The listing builds one solid part. Answer for the finished solid, in the listing's coordinates (mm). Face numbers are marked on the shaded views. A direction names the side the tool comes from. Round coordinates to 2 decimals unless told otherwise and drop trailing zeros. Loops run counter-clockwise (first coordinate to the right, second up) from the corner with the lowest first, then second, coordinate; pieces in that order, holes last. Notation, with made-up numbers: M 38,43.5 L 52,43.5 A14 cw 52,57.5 Z; hole C -12,64 d6. An arc over 180 degrees is marked long. Answer as a JSON object with one key per item and string values.
```python
from build123d import *

# Parameters (mm, degrees)
SKETCH1_W           = 70
SKETCH1_H           = 100
BOSS_EXTRUDE1_DEPTH = 40
SKETCH2_W           = 66
SKETCH2_H           = 92
CUT_EXTRUDE1_DEPTH  = 33
SKETCH3_W           = 4
SKETCH3_H           = 92
CUT_EXTRUDE2_DEPTH  = 71
SKETCH4_R           = 10.75
CUT_EXTRUDE3_DEPTH  = 3.5
CUT_EXTRUDE4_DEPTH  = 5.5
SKETCH6_R           = 1.1
CUT_EXTRUDE5_DEPTH  = 3
SKETCH11_W          = 10
SKETCH11_H          = 92
CUT_EXTRUDE9_DEPTH  = 10
SKETCH12_W          = 2.25
SKETCH12_H          = 40
CUT_EXTRUDE10_DEPTH = 5
SKETCH13_W          = 2.25
SKETCH13_H          = 40
CUT_EXTRUDE11_DEPTH = 5
SKETCH16_R          = 11.75
BOSS_EXTRUDE3_DEPTH = 8.5
SKETCH17_R          = 10.7
CUT_EXTRUDE13_DEPTH = 10
SKETCH19_W          = 20.5
SKETCH19_H          = 10.2
CUT_EXTRUDE14_DEPTH = 101


with BuildPart() as part:
    # Sketch1 → Boss-Extrude1 (new body)
    with BuildSketch(Plane.XY):
        Rectangle(SKETCH1_W, SKETCH1_H)
    extrude(amount=BOSS_EXTRUDE1_DEPTH)

    # Sketch2 → Cut-Extrude1 (cut)
    with BuildSketch(Plane.XY.offset(40)):
        Rectangle(SKETCH2_W, SKETCH2_H)
    extrude(amount=-CUT_EXTRUDE1_DEPTH, mode=Mode.SUBTRACT)

    # Sketch3 → Cut-Extrude2 (cut, through all)
    with BuildSketch(Plane.ZY.offset(35)):
        with Locations((6.5, 0)):
            Rectangle(SKETCH3_W, SKETCH3_H)
    extrude(amount=-CUT_EXTRUDE2_DEPTH, mode=Mode.SUBTRACT)

    # Sketch4 → Cut-Extrude3 (cut)
    with BuildSketch(Plane(origin=(0, 0, 0), x_dir=(-1, 0, 0), z_dir=(0, 0, -1))):
        Circle(SKETCH4_R)
    extrude(amount=-CUT_EXTRUDE3_DEPTH, mode=Mode.SUBTRACT)

    # Sketch5 → Cut-Extrude4 (cut, through all)
    with BuildSketch(Plane.XY.offset(4.5)):
        Polygon((-15.010107583, -6), (-35.010107583, -6), (-35.010107583, 6), (-28.010107583, 6), (-22.010107583, 6), (-15.010107583, 6), align=None)
        Polygon((15.010107583, -6), (35.010107583, -6), (35.010107583, 6), (28.010107583, 6), (22.010107583, 6), (15.010107583, 6), align=None)
    extrude(amount=-CUT_EXTRUDE4_DEPTH, mode=Mode.SUBTRACT)

    # Sketch6 → Cut-Extrude5 (cut)
    with BuildSketch(Plane.XZ.offset(50)):
        with Locations((27, 8.9)):
            Circle(SKETCH6_R)
        with Locations((27, 17.4)):
            Circle(SKETCH6_R)
        with Locations((-27, 8.9)):
            Circle(SKETCH6_R)
        with Locations((-27, 17.4)):
            Circle(SKETCH6_R)
    extrude(amount=-CUT_EXTRUDE5_DEPTH, mode=Mode.SUBTRACT)

    # Sketch11 → Cut-Extrude9 (cut)
    with BuildSketch(Plane.XY.offset(4.5)):
        with Locations((-30, 0)):
            Rectangle(SKETCH11_W, SKETCH11_H)
        with Locations((30, 0)):
            Rectangle(SKETCH11_W, SKETCH11_H)
    extrude(amount=-CUT_EXTRUDE9_DEPTH, mode=Mode.SUBTRACT)

    # Sketch12 → Cut-Extrude10 (cut)
    with BuildSketch(Plane(origin=(25, 0, 0), x_dir=(0, 0, -1), z_dir=(1, 0, 0))):
        with Locations((-1.125, -26)):
            Rectangle(SKETCH12_W, SKETCH12_H)
    extrude(amount=-CUT_EXTRUDE10_DEPTH, mode=Mode.SUBTRACT)

    # Sketch13 → Cut-Extrude11 (cut)
    with BuildSketch(Plane.ZY.offset(25)):
        with Locations((1.125, -26)):
            Rectangle(SKETCH13_W, SKETCH13_H)
    extrude(amount=-CUT_EXTRUDE11_DEPTH, mode=Mode.SUBTRACT)

    # Sketch16 → Boss-Extrude3 (add)
    with BuildSketch(Plane(origin=(0, 0, 0), x_dir=(-1, 0, 0), z_dir=(0, 0, -1))):
        Circle(SKETCH16_R)
    extrude(amount=BOSS_EXTRUDE3_DEPTH)

    # Sketch17 → Cut-Extrude13 (cut)
    with BuildSketch(Plane(origin=(0, 0, -8.5), x_dir=(-1, 0, 0), z_dir=(0, 0, -1))):
        Circle(SKETCH17_R)
    extrude(amount=-CUT_EXTRUDE13_DEPTH, mode=Mode.SUBTRACT)

    # Sketch19 → Cut-Extrude14 (cut, through all)
    with BuildSketch(Plane(origin=(0, 50, 0), x_dir=(1, 0, 0), z_dir=(0, 1, 0))):
        with Locations((0, -9.6)):
            Rectangle(SKETCH19_W, SKETCH19_H)
    extrude(amount=-CUT_EXTRUDE14_DEPTH, mode=Mode.SUBTRACT)


solid = part.part
```
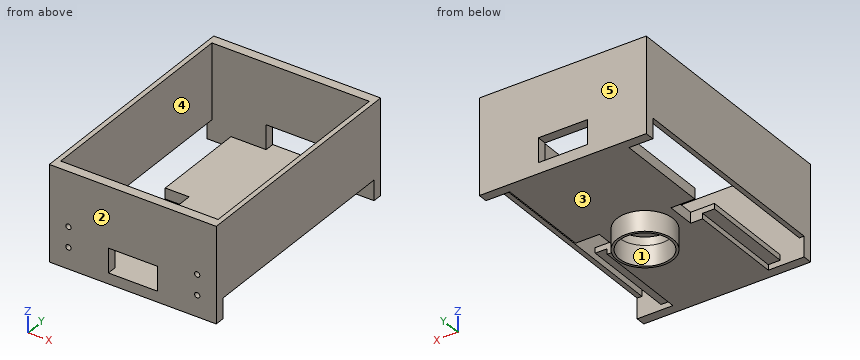
Item 1: The part is cut by section B-B (z = 6). Give the vertices of the cut face in (x, y), then the cut area to 3 significant figures.
Values follow:
{"outline": "M -35,-50 L -10.25,-50 L -10.25,-46 L -35,-46 Z; M -35,46 L -10.25,46 L -10.25,50 L -35,50 Z; M 10.25,-50 L 35,-50 L 35,-46 L 10.25,-46 Z; M 10.25,46 L 35,46 L 35,50 L 10.25,50 Z", "area": "396 mm^2"}
Item 2: The part is cut by section D-D (z = 34). Give the vertices of the cut face in (x, y), then the cut area to 3 significant figures.
Values follow:
{"outline": "M -35,-50 L 35,-50 L 35,50 L -35,50 Z; hole M -33,-46 L 33,-46 L 33,46 L -33,46 Z", "area": "928 mm^2"}
Item 3: Flat-ended cylindrical pins translate along their axes: P1, Ø12, axis at x = 18, y = 31.5, coming from the +Z side; P2, Ø3, axis at x = -1, y = 47.5, coming from the -Z side; P3, Ø2.5, axis at x = 23, y = -19, coming from the -Z side; P4, Ø2.5, axis at x = -27, z = 17, coming from the -Y side. Find the tip coordinate at first contact, or state that the pin passes through.
Values follow:
{"P1": "z = 4.5", "P2": "z = 0", "P3": "z = 2.25", "P4": "y = -50"}
Item 4: Which of the six approach directions +Z, -Z, +X, -X, +Y, -Y give full straight-line access (tool end or side, diameter ignored) to the marked faces 1 and 2?
Values follow:
{"face 1": "-Z", "face 2": "+Z, -Z, +X, -X, -Y"}
Item 5: Straight lines are drawn through the part: line 1 (Z direction, x = -27, y = -47.75); line 2 (X direction, y = 18.5, z = 34); line 3 (Y direction, x = -23.5, z = 3.5). For each, find the intervals that lie inside material, in ascending order.
Values follow:
{"line 1": "0 to 7.8, 10 to 16.3, 18.5 to 40", "line 2": "-35 to -33, 33 to 35", "line 3": "-50 to -6, 6 to 50"}
Item 6: The part is cut by section A-A (y = 0). Give the vertices of the cut face in (x, z), then the cut area to 3 significant figures.
Values follow:
{"outline": "M -35,8.5 L -33,8.5 L -33,40 L -35,40 Z; M -15.01,0 L -11.75,0 L -11.75,-8.5 L -10.7,-8.5 L -10.7,0 L -10.75,0 L -10.75,3.5 L 10.75,3.5 L 10.75,0 L 10.7,0 L 10.7,-8.5 L 11.75,-8.5 L 11.75,0 L 15.01,0 L 15.01,4.5 L -15.01,4.5 Z; M 33,8.5 L 35,8.5 L 35,40 L 33,40 Z", "area": "204 mm^2"}
Item 7: Determine the mould class of the marked faces 3, 4 and 5 for opening direction Y: released by +Y, released by -Y, zero draft, split by the parting line, or undercut.
Values follow:
{"face 3": "zero draft", "face 4": "undercut", "face 5": "released by +Y"}
Item 8: The part is cut by section C-C (x = 22). Give the vertices of the cut face in (y, z).
Values follow:
{"outline": "M -50,0 L -46,0 L -46,2.25 L -6,2.25 L -6,4.5 L -46,4.5 L -46,40 L -50,40 Z; M 6,0 L 50,0 L 50,40 L 46,40 L 46,4.5 L 6,4.5 Z"}
